Autodesk Inventor part; units mm, degrees
ref_plane "YZ Plane" through (0, 0, 0) normal (1, 0, 0) x (0, 1, 0)
ref_plane "XZ Plane" through (0, 0, 0) normal (0, 1, 0) x (-1, 0, 0)
ref_plane "XY Plane" through (0, 0, 0) normal (0, 0, 1) x (1, 0, 0)
sketch "Sketch1" plane through (0, 0, 0) normal (0, 1, 0) x (-1, 0, 0)
  line L0 (0, 0) -> (25.4, 0)
  line L1 (25.4, 0) -> (25.4, 25.4)
  line L2 (25.4, 25.4) -> (0, 25.4)
  line L3 (0, 25.4) -> (0, 0)
  line L4 (1.5875, 23.8125) -> (23.8125, 23.8125)
  line L5 (23.8125, 23.8125) -> (23.8125, 1.5875)
  line L6 (23.8125, 1.5875) -> (1.5875, 1.5875)
  line L7 (1.5875, 1.5875) -> (1.5875, 23.8125)
  dimension "d0" = 25.4
  dimension "d2" = 25.4
  dimension "d3" = 1.5875
extrude "Extrusion1" add sketch "Sketch1" along normal blind 120.65
sketch "Sketch2" plane through (-25.4, 0, 0) normal (-1, 0, 0) x (0, 0, 1)
  line L0 (0, 0) -> (25.4, 0)
  line L1 (0, 0) -> (0, 120.65)
  line L2 (25.4, 0) -> (0, 25.4)
  dimension "d6" = 45
extrude "Extrusion2" cut sketch "Sketch2" against normal blind 25.4
sketch "Sketch3" plane through (-25.4, 120.65, 0) normal (-1, 0, 0) x (0, 0, 1)
  circle A0 centre (12.7, -95.25) radius 3.3782
  circle A1 centre (12.7, -57.15) radius 3.3782
  point P0 (0, -120.65)
extrude "Extrusion3" cut sketch "Sketch3" against normal blind 25.4
sketch "Sketch4" plane through (-25.4, 120.65, 25.4) normal (0, 0, 1) x (1, 0, 0)
  circle A0 centre (12.7, -12.7) radius 3.3782
  circle A1 centre (12.7, -12.7) radius 3.3782
extrude "Extrusion4" cut sketch "Sketch4" against normal blind 25.4
properties part number "Square Tube 6" material "Aluminum 6061"
Geometry check sheet. Reference: the model listing, model coordinates, mm. A direction names the side the tool comes from. Give positions to 0.01 mm unless a question says otherwise; leave off trailing zeros. Write each loop counter-clockwise with the first axis right and the second up, starting at its lowest first coordinate (ties: lowest second). Pieces come first, ordered by that corner, then holes. Notation, with made-up numbers: (12, 10) -> (41, 10) arc R18 ccw to (41, 33) -> close; hole circle Ø5 at (59.5, -22). An arc over 180 degrees is marked (long way). Use one line per item in the form item = value.
Item 1: Depth check by flat-ended pin: pin 1 Ø10 at (x, z) = (-11, 14) entering from +Y. Enter the tip coordinate at first touch or a pass-through.
Results list:
pin_1 = through
Item 2: Sectioned sample at D-D on y = 63.5. Enter the section's corners in (x, z), plus the area to 3 significant figures.
Results list:
outline = (-25.4, 0) -> (0, 0) -> (0, 9.32) -> (-1.59, 9.32) -> (-1.59, 1.59) -> (-23.81, 1.59) -> (-23.81, 9.32) -> (-25.4, 9.32) -> close; (-25.4, 16.08) -> (-23.81, 16.08) -> (-23.81, 23.81) -> (-1.59, 23.81) -> (-1.59, 16.08) -> (0, 16.08) -> (0, 25.4) -> (-25.4, 25.4) -> close
area = 130 mm2
Item 3: Access from +Z, -Z, +X, -X, +Y, -Y to the whole of each face (thin tool, end or side, straight path). Record for faces 1 (the flat face through (-13, 60, 23.812)), 2 (the flat face through (-13, 72, 0)).
Results list:
face_1 = +Y, -Y
face_2 = -Z, +X, -X, +Y, -Y
Item 4: Sectioned sample at B-B on z = 12.7. Enter the section's corners in (x, y).
Results list:
outline = (-25.4, 12.7) -> (-23.81, 12.7) -> (-23.81, 22.02) -> (-25.4, 22.02) -> close; (-25.4, 28.78) -> (-23.81, 28.78) -> (-23.81, 60.12) -> (-25.4, 60.12) -> close; (-25.4, 66.88) -> (-23.81, 66.88) -> (-23.81, 120.65) -> (-25.4, 120.65) -> close; (-1.59, 12.7) -> (0, 12.7) -> (0, 22.02) -> (-1.59, 22.02) -> close; (-1.59, 28.78) -> (0, 28.78) -> (0, 60.12) -> (-1.59, 60.12) -> close; (-1.59, 66.88) -> (0, 66.88) -> (0, 120.65) -> (-1.59, 120.65) -> close
Item 5: Sectioned sample at C-C on x = -12.7. Enter the section's corners in (y, z), plus the area to 3 significant figures.
Results list:
outline = (0, 25.4) -> (1.59, 23.81) -> (104.57, 23.81) -> (104.57, 25.4) -> close; (23.81, 1.59) -> (25.4, 0) -> (104.57, 0) -> (104.57, 1.59) -> close; (111.33, 0) -> (120.65, 0) -> (120.65, 1.59) -> (111.33, 1.59) -> close; (111.33, 23.81) -> (120.65, 23.81) -> (120.65, 25.4) -> (111.33, 25.4) -> close
area = 321 mm2
Item 6: Mould release check, pull along Y, two halves, no side actions. Record for faces 3 (the flat face through (-24, 12.6, 12.8)), 4 (the cylindrical face through (-24.62, 60.2, 11.97)), 5 (the flat face through (-13, 72, 1.588)): released by +Y, released by -Y, zero draft, split by the parting line, or undercut.
Results list:
face_3 = released by -Y
face_4 = undercut
face_5 = zero draft
Item 7: Scan lines: line 1 (X direction, y = 36, z = 21.25); line 2 (Y direction, x = -0.45, z = 12.7); line 3 (Z direction, x = -12.25, y = 70). Record each from-to range of solid material in increasing order.
Results list:
line_1 = -25.4 to -23.81, -1.59 to 0
line_2 = 12.7 to 22.02, 28.78 to 60.12, 66.88 to 120.65
line_3 = 0 to 1.59, 23.81 to 25.4
Item 8: Sectioned sample at A-A on y = 101. Enter the section's corners in (x, z).
Results list:
outline = (-25.4, 0) -> (0, 0) -> (0, 25.4) -> (-25.4, 25.4) -> close; hole (-23.81, 1.59) -> (-1.59, 1.59) -> (-1.59, 23.81) -> (-23.81, 23.81) -> close
